Verification items for this drawing (mm, ordinates from the low corner). Give positions to 0.01 mm unless a question says otherwise; leave off trailing zeros. Write each loop counter-clockwise with the first axis right and the second up, starting at its lowest first coordinate (ties: lowest second). Pieces come first, ordered by that corner, then holes. Notation, with made-up numbers: M -13.75,-32 L -6.75,-32 A20 ccw -6.75,-22 Z; hole C -14,46.25 d3. An arc over 180 degrees is marked long. Use one line per item in the form item = value. Start each with the question number.
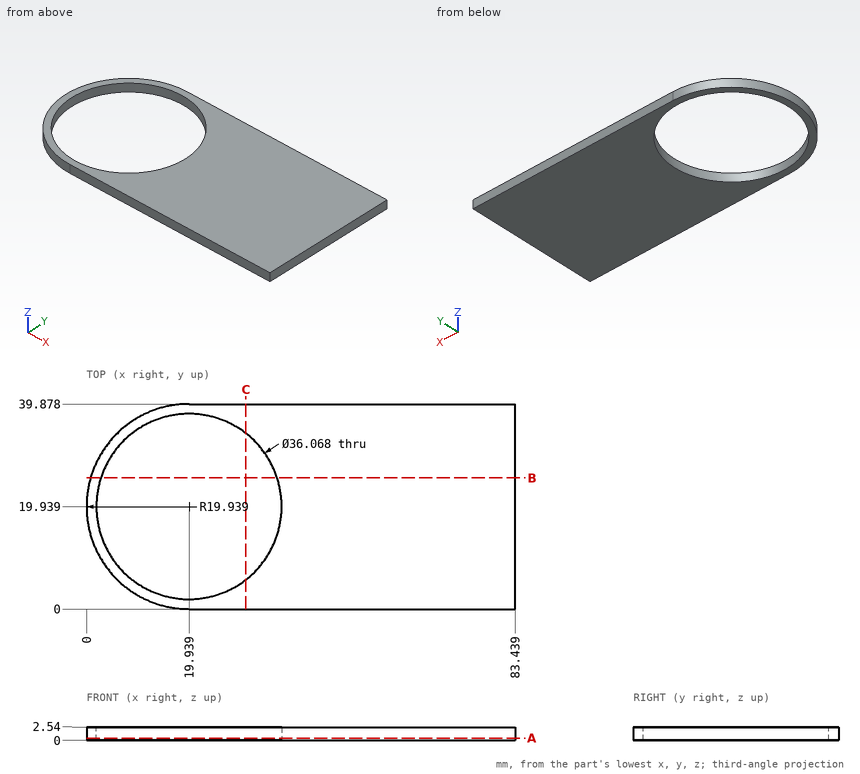
(1) Depth check by flat-ended pin: pin 1 (1 mm diameter, centred on x = 34.5, y = 7, fed in from -Z). Enter the tip coordinate at first touch or a pass-through.
(2) Sectioned sample at C-C, the plane x = 31. Record the boundary of the cut face in (y, z), plus the area to 3 significant figures.
(3) Sectioned sample at B-B, the plane y = 25.5. Record the boundary of the cut face in (x, z).
(4) Thickness scan on probe 1 along X at (y, z) = (20, 2.05); probe 2 along Y at (x, z) = (19, 1.5); probe 3 along X at (y, z) = (12, 1.25). Record the ranges inside material, lowest first. Write a range as [from, to].
(5) Sectioned sample at A-A, the plane z = 0.4. Record the boundary of the cut face in (x, y).
Numbers:
q1.pin_1 = 0
q2.outline = M 0,0 L 5.7,0 L 5.7,2.54 L 0,2.54 Z; M 34.18,0 L 39.88,0 L 39.88,2.54 L 34.18,2.54 Z
q2.area = 28.9 mm2
q3.outline = M 0.79,0 L 2.78,0 L 2.78,2.54 L 0.79,2.54 Z; M 37.09,0 L 83.44,0 L 83.44,2.54 L 37.09,2.54 Z
q4.probe_1 = [0, 1.91], [37.97, 83.44]
q4.probe_2 = [0.02, 1.93], [37.95, 39.86]
q4.probe_3 = [1.65, 3.75], [36.13, 83.44]
q5.outline = M 19.94,0 L 83.44,0 L 83.44,39.88 L 19.94,39.88 A19.94 ccw Z; hole C 19.94,19.94 d36.07
